Drawing for the job (mm, zero at the part's lowest x, y, z). A direction names the side the tool comes from. Round coordinates to 2 decimals unless told otherwise and drop trailing zeros. Write each loop counter-clockwise with the first axis right and the second up, starting at its lowest first coordinate (ties: lowest second). Pieces come first, ordered by that corner, then holes. Notation, with made-up numbers: M -29,32 L 12,32 A18 ccw 12,43 Z; hole C 14,76.5 d6. An arc over 180 degrees is marked long. Use a Markdown table: item, result.
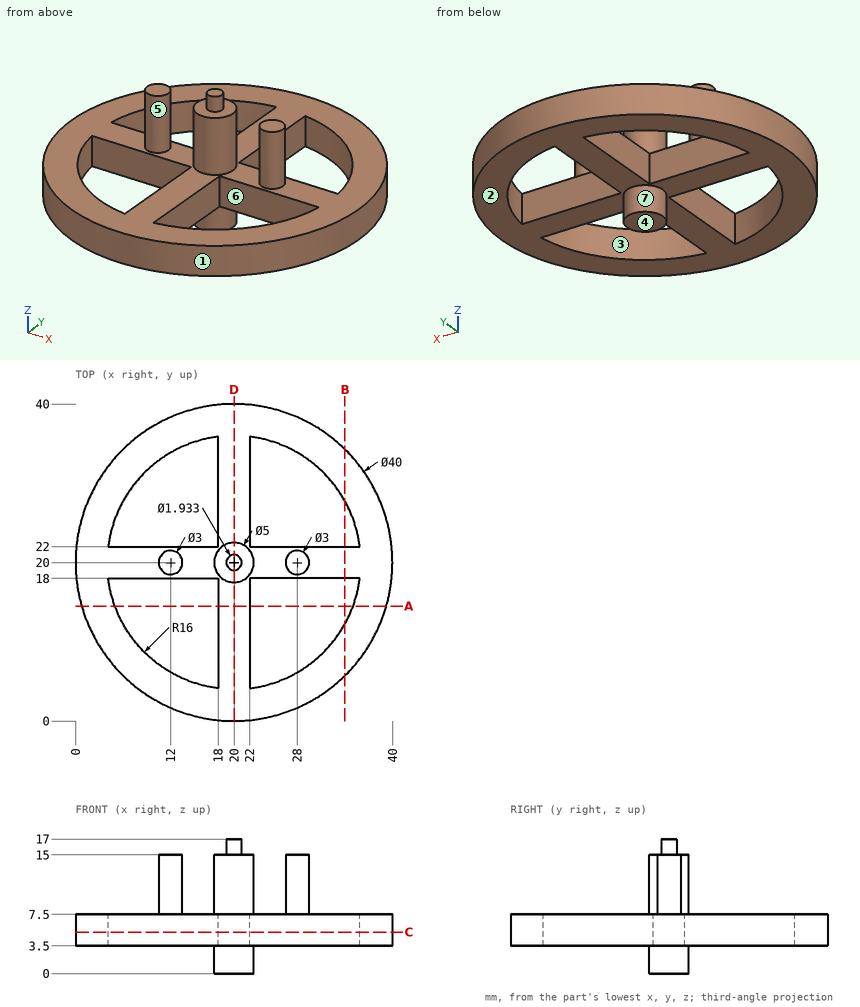
Q1. Cut at A-A on y = 14.5. Give the cut face in (x, z) (3 decimals).
Response values:
| item | result |
|---|---|
| outline | M 0.771,3.5 L 4.975,3.5 L 4.975,7.5 L 0.771,7.5 Z; M 18,3.5 L 22,3.5 L 22,7.5 L 18,7.5 Z; M 35.025,3.5 L 39.229,3.5 L 39.229,7.5 L 35.025,7.5 Z |
Q2. Drill centre lines: L1, parallel to X at y = 28, z = 5.25; L2, parallel to Y at x = 24, z = 5; L3, parallel to X at y = 26, z = 5.5. Where is each one in solid material? Low to high.
Response values:
| item | result |
|---|---|
| L1 | x = 1.67 to 6.14, 18 to 22, 33.86 to 38.33 |
| L2 | y = 0.4 to 4.51, 18 to 22, 35.49 to 39.6 |
| L3 | x = 0.92 to 5.17, 18 to 22, 34.83 to 39.08 |
Q3. Which spindle directions (+Z, -Z, +X, -X, +Y, -Y) get a long thin tool onto all of the face, cutting with end or side? Do the marked faces 4, 5, 6 and 7. Say none if no direction does.
Response values:
| item | result |
|---|---|
| face 4 | -Z, +X, -X, +Y, -Y |
| face 5 | +Z |
| face 6 | +Z, -Z |
| face 7 | -Z |
Q4. Cut at C-C on z = 5.25. Give the cut face in (x, y), and give its area (3 significant figures).
Response values:
| item | result |
|---|---|
| outline | C 20,20 d40; hole M 4.13,18 A16 ccw 18,4.13 L 18,18 Z; hole M 4.13,22 L 18,22 L 18,35.87 A16 ccw Z; hole M 22,4.13 A16 ccw 35.87,18 L 22,18 Z; hole M 22,22 L 35.87,22 A16 ccw 22,35.87 Z |
| area | 692 mm2 |
Q5. Cut at B-B on x = 34. Give the cut face in (y, z).
Response values:
| item | result |
|---|---|
| outline | M 5.72,3.5 L 12.25,3.5 L 12.25,7.5 L 5.72,7.5 Z; M 18,3.5 L 22,3.5 L 22,7.5 L 18,7.5 Z; M 27.75,3.5 L 34.28,3.5 L 34.28,7.5 L 27.75,7.5 Z |
Q6. Cut at D-D on x = 20. Give the cut face in (y, z), and give its area (3 significant figures).
Response values:
| item | result |
|---|---|
| outline | M 0,3.5 L 17.5,3.5 L 17.5,0 L 22.5,0 L 22.5,3.5 L 40,3.5 L 40,7.5 L 22.5,7.5 L 22.5,15 L 20.97,15 L 20.97,17 L 19.03,17 L 19.03,15 L 17.5,15 L 17.5,7.5 L 0,7.5 Z |
| area | 219 mm2 |
Q7. Drop flat-ended pins along their axis: P1, Ø0.9, axis at x = 28, y = 20.5, coming from the +Z side; P2, Ø1.2, axis at x = 29.5, z = 6, coming from the +Y side; P3, Ø1.2, axis at y = 28.5, z = 5, coming from the -X side. Give the stop position or say it passes through.
Response values:
| item | result |
|---|---|
| P1 | stops at z = 15 |
| P2 | stops at y = 37.91 |
| P3 | stops at x = 1.63 |
Q8. Two-plate mould, pull along X, no slides. Class the marked faces 1, 2 and 3: +X half, -X half, draft (parallel to the pull), parting line (faces both ways), or undercut.
Response values:
| item | result |
|---|---|
| face 1 | parting line |
| face 2 | draft |
| face 3 | undercut |
